from build123d import *

# Parameters (mm, degrees)
SKETCH_2_R                    = 1.5
EXTRUDE_1_DEPTH               = 24
CHAMFER_1_SIZE                = 0.1
SKETCH_3_W                    = 2.5
SKETCH_3_H                    = 0.5
CUT_EXTRUDE_1_DEPTH           = 0.5
CUT_EXTRUDE_1_DRAFT           = -10
SKETCH_3_W_2                  = 0.5
SKETCH_3_H_2                  = 2.5
CUT_EXTRUDE_1_PROFILE_2_DEPTH = 0.5
CUT_EXTRUDE_1_PROFILE_2_DRAFT = -10
FILLET_1_R                    = 0.3


with BuildPart() as part:
    # 草图1 → 旋转1 (revolve)
    with BuildSketch(Plane.XY, mode=Mode.PRIVATE) as revolve_1_sk:
        Polygon((0, 0), (2.5, 0), (1.5, -0.8), (0, -0.8), align=None)
    revolve(revolve_1_sk.sketch.rotate(Axis((0, -0.8, 0), (0, 1, 0)), 90), axis=Axis((0, -0.8, 0), (0, 1, 0)))

    # 草图2 → 凸台-拉伸1 (add)
    with BuildSketch(Plane.XZ.offset(0.8)):
        with Locations(Location((0, 0, 0), (0, 0, 270))):
            Circle(SKETCH_2_R)
    extrude(amount=EXTRUDE_1_DEPTH)

    # 倒角1
    chamfer_1_edges = [part.edges().sort_by_distance(p)[0] for p in [
        (0, -24.8, 1.5),
    ]]
    chamfer(chamfer_1_edges, length=CHAMFER_1_SIZE)


with BuildPart() as cut_extrude_1_tool:
    # 草图3 → 切除-拉伸1 (with draft: the straight prism first)
    with BuildSketch(Plane(origin=(0, 0, 0), x_dir=(1, 0, 0), z_dir=(0, 1, 0))):
        Rectangle(SKETCH_3_W, SKETCH_3_H)
    extrude(amount=-CUT_EXTRUDE_1_DEPTH)
    # 切除-拉伸1: the draft: its side faces are tilted about the plane it starts from
    cut_extrude_1_sides = [cut_extrude_1_tool.faces().sort_by_distance(p)[0] for p in [
        (0, -0.25, 0.25),
        (1.25, -0.25, 0),
        (0, -0.25, -0.25),
        (-1.25, -0.25, 0),
    ]]
    draft(cut_extrude_1_sides, Plane(origin=(0, 0, 0), x_dir=(1, 0, 0), z_dir=(0, 1, 0)), CUT_EXTRUDE_1_DRAFT)


with BuildPart() as part_1:
    add(part.part)

    # 切除-拉伸1: cut by cut_extrude_1_tool
    add(cut_extrude_1_tool.part, mode=Mode.SUBTRACT)


with BuildPart() as cut_extrude_1_profile_2_tool:
    # 草图3 → 切除-拉伸1 profile 2 (with draft: the straight prism first)
    with BuildSketch(Plane(origin=(0, 0, 0), x_dir=(1, 0, 0), z_dir=(0, 1, 0))):
        Rectangle(SKETCH_3_W_2, SKETCH_3_H_2)
    extrude(amount=-CUT_EXTRUDE_1_PROFILE_2_DEPTH)
    # 切除-拉伸1 profile 2: the draft: its side faces are tilted about the plane it starts from
    cut_extrude_1_profile_2_sides = [cut_extrude_1_profile_2_tool.faces().sort_by_distance(p)[0] for p in [
        (-0.25, -0.25, 0),
        (0, -0.25, 1.25),
        (0.25, -0.25, 0),
        (0, -0.25, -1.25),
    ]]
    draft(cut_extrude_1_profile_2_sides, Plane(origin=(0, 0, 0), x_dir=(1, 0, 0), z_dir=(0, 1, 0)), CUT_EXTRUDE_1_PROFILE_2_DRAFT)


with BuildPart() as part_2:
    add(part_1.part)

    # 切除-拉伸1 profile 2: cut by cut_extrude_1_profile_2_tool
    add(cut_extrude_1_profile_2_tool.part, mode=Mode.SUBTRACT)

    # 圆角1
    fillet_1_edges = [part_2.edges().sort_by_distance(p)[0] for p in [
        (0.205918255, -0.25, -0.205918255),
        (0.205918255, -0.25, 0.205918255),
        (-0.205918255, -0.25, 0.205918255),
        (-0.205918255, -0.25, -0.205918255),
    ]]
    fillet(fillet_1_edges, radius=FILLET_1_R)


solid = part_2.part
Here's how the part is built. I have some questions about the finished solid (model axes, mm). Coordinates: 2 decimals unless noted, no trailing zeros. Loops run counter-clockwise (first coordinate to the right, second up) from the corner with the lowest first, then second, coordinate; pieces in that order, holes last.
1. Imagine slicing it at A-A, the plane y = -17.25. Please give me the cut outline in (x, z), and give its area (3 significant figures).
2. For P1, Ø1, axis at y = -11.5, z = 0, coming from the +X side; P2, Ø3, axis at x = 1, y = -3, coming from the +Z side, each with a flat end and sliding along its axis, tell me the tip position at first contact or that it passes through.
3. I need wall thicknesses on L1, parallel to X at y = -21.25, z = -0.1; L2, parallel to X at y = -12.5, z = 0.55; L3, parallel to Y at x = 0.5, z = 1.75. Which ranges of each line are inside material? Lowest first, please.
4. If we mould it in two halves opening along Z, with no side actions, what happens to faces 1 (the flat face through (0, -24.8, 0)), 2 (the flat face through (0, -0.5, 0)), 3 (the cylindrical face through (0.45, -12.58, -1.43))? For each: pulls with the +Z half, pulls with the -Z half, needs draft (parallel to the pull), parting line crosses it, or undercut.
Taken from the geometry:
1. outline: circle Ø3 at (0, 0)
1. area: 7.07 mm2
2. P1: stops at x = 1.5
2. P2: stops at z = 1.5
3. L1: x = -1.5 to 1.5
3. L2: x = -1.4 to 1.4
3. L3: y = -0.54 to 0
4. face 1: needs draft
4. face 2: undercut
4. face 3: parting line crosses it
